```python
from build123d import *

# Parameters (mm, degrees)
F0_W     = 100
F0_H     = 96
F1_DEPTH = 4
F2_W     = 4
F2_H     = 4
F3_DEPTH = 4
F5_DEPTH = 4


with BuildPart() as f1:
    # F0 (on Top) → F1 (new body)
    with BuildSketch(Plane.XY):
        with Locations((-50, 48)):
            Rectangle(F0_W, F0_H)
    extrude(amount=F1_DEPTH)

    # F2 (on face) → F3 (cut, through all)
    with BuildSketch(Plane.XY.offset(4)):
        with Locations((-2, 2)):
            Rectangle(F2_W, F2_H)
        with Locations((-10, 2)):
            Rectangle(F2_W, F2_H)
        with Locations((-2, 94)):
            Rectangle(F2_W, F2_H)
        with Locations((-10, 94)):
            Rectangle(F2_W, F2_H)
        with Locations((-98, 94)):
            Rectangle(F2_W, F2_H)
        with Locations((-90, 2)):
            Rectangle(F2_W, F2_H)
        with Locations((-98, 2)):
            Rectangle(F2_W, F2_H)
        with Locations((-90, 94)):
            Rectangle(F2_W, F2_H)
    extrude(amount=-F3_DEPTH, mode=Mode.SUBTRACT)

    # F4 (on face) → F5 (cut, through all)
    with BuildSketch(Plane.XY.offset(4)):
        with BuildLine():
            ThreePointArc((-85, 23), (-82.071068, 15.928932), (-75, 13))
            Line((-75, 13), (-25, 13))
            ThreePointArc((-25, 13), (-17.928932, 15.928932), (-15, 23))
            Line((-15, 23), (-15, 73))
            ThreePointArc((-15, 73), (-17.928932, 80.071068), (-25, 83))
            Line((-25, 83), (-75, 83))
            ThreePointArc((-75, 83), (-82.071068, 80.071068), (-85, 73))
            Line((-85, 73), (-85, 23))
        make_face()
    extrude(amount=-F5_DEPTH, mode=Mode.SUBTRACT)


solid = f1.part
```
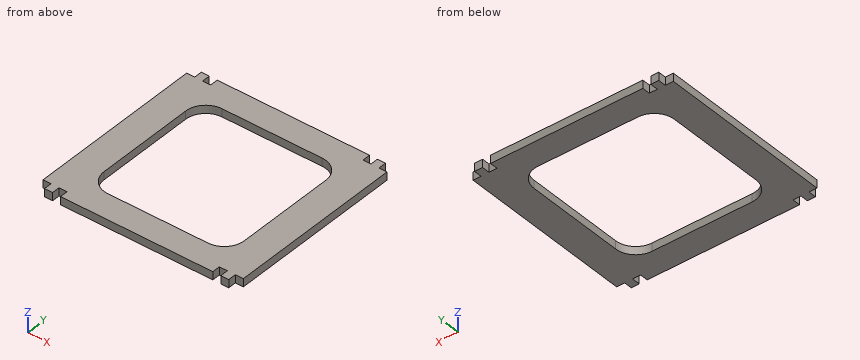
Here's how the part is built. I have some questions about the finished solid (model axes, mm). Round coordinates to 2 decimals unless told otherwise and drop trailing zeros. Write each loop counter-clockwise with the first axis right and the second up, starting at its lowest first coordinate (ties: lowest second). Pieces come first, ordered by that corner, then holes.
Q1. If we section it at C-C on x = -10.5: Write out the boundary of the cut face in (y, z), plus the area to 3 significant figures.
Q2. If we section it at A-A on y = 81: Write out the boundary of the cut face in (x, z).
Q3. Please list where these lines run through material, in increasing order: probe 1 along X at (y, z) = (92.5, 1.5); probe 2 along X at (y, z) = (64, 1.4); probe 3 along Y at (x, z) = (-33, 3.3).
Q4. If we section it at B-B on x = -57: Write out the boundary of the cut face in (y, z), plus the area to 3 significant figures.
Q5. Will these pins go through, and if not, where does the flat tip stop? P1, Ø2, axis at y = 94.5, z = 2, coming from the +X side; P2, Ø2, axis at y = 93.5, z = 1.5, coming from the -X side; P3, Ø1.2, axis at x = -89.5, z = 1.5, coming from the -Y side.
Answer below:
1. outline: (4, 0) - (92, 0) - (92, 4) - (4, 4) - close
1. area: 352 mm2
2. outline: (-100, 0) - (-81, 0) - (-81, 4) - (-100, 4) - close; (-19, 0) - (0, 0) - (0, 4) - (-19, 4) - close
3. probe 1: x = -96 to -92, -88 to -12, -8 to -4
3. probe 2: x = -100 to -85, -15 to 0
3. probe 3: y = 0 to 13, 83 to 96
4. outline: (0, 0) - (13, 0) - (13, 4) - (0, 4) - close; (83, 0) - (96, 0) - (96, 4) - (83, 4) - close
4. area: 104 mm2
5. P1: stops at x = -4
5. P2: stops at x = -96
5. P3: stops at y = 4
